The model under review builds one solid part; all positions refer to its coordinate system, in mm. Coordinates: 2 decimals unless noted, no trailing zeros. Write each loop counter-clockwise with the first axis right and the second up, starting at its lowest first coordinate (ties: lowest second). Pieces come first, ordered by that corner, then holes.
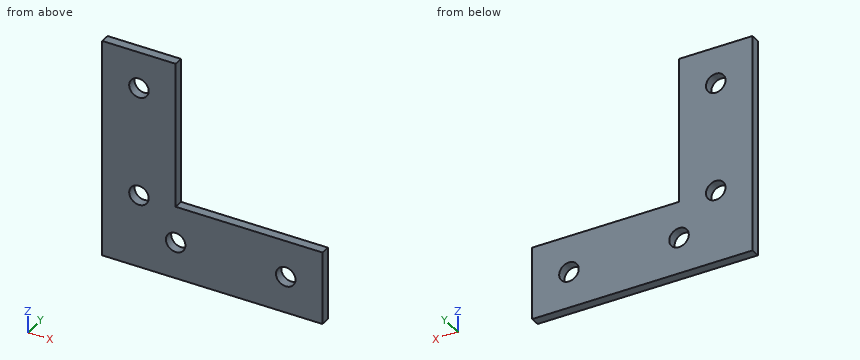
Autodesk Inventor part; units mm, degrees
ref_plane "YZ Plane" through (0, 0, 0) normal (1, 0, 0) x (0, 1, 0)
ref_plane "XZ Plane" through (0, 0, 0) normal (0, 1, 0) x (-1, 0, 0)
ref_plane "XY Plane" through (0, 0, 0) normal (0, 0, 1) x (1, 0, 0)
sketch "Sketch1" plane through (0, 0, 0) normal (0, 1, 0) x (-1, 0, 0)
  circle A0 centre (-63.5, 12.7) radius 3.3782
  circle A1 centre (-25.4, 12.7) radius 3.3782
  circle A2 centre (-12.7, 25.4) radius 3.3782
  circle A3 centre (-12.7, 63.5) radius 3.3782
  line L0 (0, 76.2) -> (0, 25.4)
  line L1 (-25.4, 76.2) -> (0, 76.2)
  line L2 (-25.4, 25.4) -> (-25.4, 76.2)
  line L3 (-76.2, 25.4) -> (-25.4, 25.4)
  line L4 (-76.2, 0) -> (-76.2, 25.4)
  line L5 (-28.829, 0) -> (-76.2, 0)
  line L6 (15.621, -25.4) -> (-28.829, -25.4)
  line L7 (-28.829, -25.4) -> (-28.829, 0)
  line L8 (0, 25.4) -> (15.621, 25.4)
  line L9 (15.621, 25.4) -> (15.621, -25.4)
  line L10 (15.621, -25.4) -> (15.621, -25.4)
  point P0 (0, 0)
  point P1 (0, 0)
  dimension "d32" = 15.621
  dimension "d44" = 50.8
extrude "Plate1" add sketch "Sketch1" along normal blind 3.175
sketch "Sketch7" plane through (0, 0, 0) normal (0, -1, 0) x (1, 0, 0)
  line L0 (28.829, -25.4) -> (-15.621, -25.4)
  line L1 (28.829, 0) -> (28.829, -25.4)
  line L2 (76.2, 0) -> (28.829, 0)
  line L3 (-15.621, 25.4) -> (0, 25.4)
  line L4 (0, 25.4) -> (0, 0)
  line L5 (0, 0) -> (28.829, 0)
  line L6 (-15.621, -25.4) -> (-15.621, 25.4)
extrude "Cut3" cut sketch "Sketch7" against normal blind 3.175
equation "\"d45\" = Thickness"
equation "\"BendRadius\" = Thickness"
equation "\"BendReliefWidth\" = Thickness"
equation "\"BendReliefDepth\" = 0.5 * Thickness"
equation "\"CornerReliefSize\" = 4 * Thickness"
equation "\"MinimumRemnant\" = 2 * Thickness"
equation "\"TransitionRadius\" = BendRadius"
equation "\"JacobiRadiusSize\" = BendRadius"
equation "\"GapSize\" = Thickness"
equation "\"d1\" = BendRadius"
properties part number "Gusset Connector 2"
Item 1: Take a section at B-B, the plane y = 1.35. Write out the cut boundary in (x, z), plus the area to 3 significant figures.
Solved:
outline: (0, 0) - (76.2, 0) - (76.2, 25.4) - (25.4, 25.4) - (25.4, 76.2) - (0, 76.2) - close; hole circle Ø6.76 at (12.7, 25.4); hole circle Ø6.76 at (12.7, 63.5); hole circle Ø6.76 at (25.4, 12.7); hole circle Ø6.76 at (63.5, 12.7)
area: 3,080 mm2
Item 2: Take a section at D-D, the plane x = 63.5. Write out the cut boundary in (y, z) (3 decimals), plus the area to 3 significant figures.
Solved:
outline: (0, 0) - (3.175, 0) - (3.175, 9.322) - (0, 9.322) - close; (0, 16.078) - (3.175, 16.078) - (3.175, 25.4) - (0, 25.4) - close
area: 59.2 mm2
Item 3: To check wall thickness, follow line 1 along Z through (x, y) = (12.7, 1.45); line 2 along Z through (x, y) = (13.5, 2.3); line 3 along X through (y, z) = (0.25, 48). State the ranges of each line that lie inside material, in increasing order.
Solved:
line 1: z = 0 to 22.02, 28.78 to 60.12, 66.88 to 76.2
line 2: z = 0 to 22.12, 28.68 to 60.22, 66.78 to 76.2
line 3: x = 0 to 25.4
Item 4: For pin 1 (1.6 mm diameter, centred on x = 43, y = 2, fed in from +Z); pin 2 (1.5 mm diameter, centred on y = 0.5, z = 64, fed in from +X), all flat-tipped, find the tip position at first contact; note any pin that passes through.
Solved:
pin 1: stops at z = 25.4
pin 2: stops at x = 25.4
Item 5: Take a section at C-C, the plane x = 12.7. Write out the cut boundary in (y, z) (3 decimals), plus the area to 3 significant figures.
Solved:
outline: (0, 0) - (3.175, 0) - (3.175, 22.022) - (0, 22.022) - close; (0, 28.778) - (3.175, 28.778) - (3.175, 60.122) - (0, 60.122) - close; (0, 66.878) - (3.175, 66.878) - (3.175, 76.2) - (0, 76.2) - close
area: 199 mm2
Item 6: Take a section at A-A, the plane z = 12.7. Write out the cut boundary in (x, y) (3 decimals), plus the area to 3 significant figures.
Solved:
outline: (0, 0) - (22.022, 0) - (22.022, 3.175) - (0, 3.175) - close; (28.778, 0) - (60.122, 0) - (60.122, 3.175) - (28.778, 3.175) - close; (66.878, 0) - (76.2, 0) - (76.2, 3.175) - (66.878, 3.175) - close
area: 199 mm2
